```python
from build123d import *

# Parameters (mm, degrees)
SKETCH_1_R      = 6.5
EXTRUDE_1_DEPTH = 5.5
SKETCH_2_R      = 4
EXTRUDE_2_DEPTH = 20
SKETCH_3_R      = 3
EXTRUDE_3_DEPTH = 11.5


with BuildPart() as part:
    # 草图1 → 凸台-拉伸1 (new body)
    with BuildSketch(Plane.XY):
        Circle(SKETCH_1_R)
    extrude(amount=-EXTRUDE_1_DEPTH)

    # 草图2 → 凸台-拉伸2 (add)
    with BuildSketch(Plane(origin=(0, 0, -5.5), x_dir=(-1, 0, 0), z_dir=(0, 0, -1))):
        Circle(SKETCH_2_R)
    extrude(amount=EXTRUDE_2_DEPTH)

    # 草图3 → 凸台-拉伸3 (add)
    with BuildSketch(Plane(origin=(0, 0, -25.5), x_dir=(-1, 0, 0), z_dir=(0, 0, -1))):
        Circle(SKETCH_3_R)
    extrude(amount=EXTRUDE_3_DEPTH)


solid = part.part
```
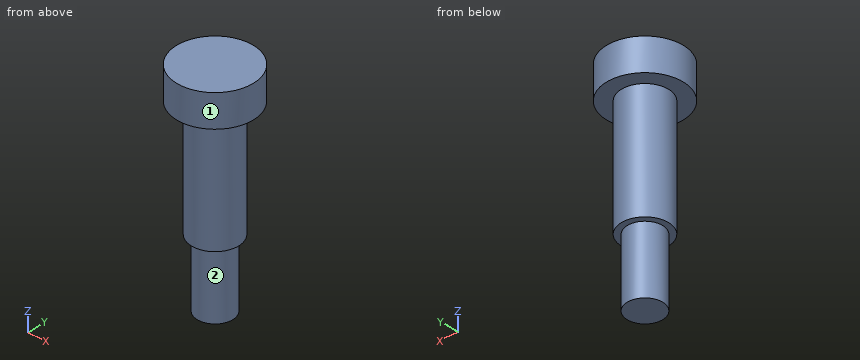
Source: CAD feature listing. Evaluate the final solid. Frame: model axes, mm. Face numbers are marked on the shaded views. A direction names the side the tool comes from. Coordinates: 2 decimals unless noted, no trailing zeros. Loops run counter-clockwise (first coordinate to the right, second up) from the corner with the lowest first, then second, coordinate; pieces in that order, holes last. Notation, with made-up numbers: (2.5, 9) -> (39.5, 9) arc R13 cw to (39.5, 22) -> close; hole circle Ø3 at (59, 30). An arc over 180 degrees is marked (long way). One line per item, written item: value. Start each with the question number.
Q1. Section query B-B, the plane x = -0.25. Return the cut outline in (y, z), and give its area (3 significant figures).
Q2. Contact query for flat-ended pins moving along their axis: P1, Ø3, axis at x = -4.5, z = -9, coming from the +Y side; P2, Ø1, axis at x = -4, z = -9.5, coming from the +Y side; P3, Ø1, axis at x = 2.5, z = -25, coming from the -Y side; P4, Ø5, axis at x = -4.5, y = 5, coming from the +Z side. Output: stop coordinate, or through.
Q3. Section query C-C, the plane z = -15.5. Return the cut outline in (x, y).
Q4. Section query D-D, the plane z = -2.5. Return the cut outline in (x, y), and give its area (3 significant figures).
Q5. Line query: line 1 along Z through (x, y) = (2, 5); line 2 along Z through (x, y) = (-1, -3.25); line 3 along X through (y, z) = (0.25, -10). Output: solid intervals per line, ascending.
Q6. Set-up query: the marked faces 1 and 2. Return all of +Z, -Z, +X, -X, +Y, -Y with unobstructed straight access to the full face (end or side cutting, diameter ignored); none if empty.
Q7. Section query A-A, the plane y = 0. Return the cut outline in (x, z).
Results:
1. outline: (-6.5, -5.5) -> (-3.99, -5.5) -> (-3.99, -25.5) -> (-2.99, -25.5) -> (-2.99, -37) -> (2.99, -37) -> (2.99, -25.5) -> (3.99, -25.5) -> (3.99, -5.5) -> (6.5, -5.5) -> (6.5, 0) -> (-6.5, 0) -> close
1. area: 300 mm^2
2. P1: y = 2.65
2. P2: y = 1.94
2. P3: y = -3.46
2. P4: z = 0
3. outline: circle Ø8 at (0, 0)
4. outline: circle Ø13 at (0, 0)
4. area: 133 mm^2
5. line 1: -5.5 to 0
5. line 2: -25.5 to 0
5. line 3: -3.99 to 3.99
6. face 1: +Z, -Z
6. face 2: -Z
7. outline: (-6.5, -5.5) -> (-4, -5.5) -> (-4, -25.5) -> (-3, -25.5) -> (-3, -37) -> (3, -37) -> (3, -25.5) -> (4, -25.5) -> (4, -5.5) -> (6.5, -5.5) -> (6.5, 0) -> (-6.5, 0) -> close
